Check sheet for the modelled part. Datum: model origin and axes. Units: mm. A direction names the side the tool comes from. Coordinates: 2 decimals unless noted, no trailing zeros. Write each loop counter-clockwise with the first axis right and the second up, starting at its lowest first coordinate (ties: lowest second). Pieces come first, ordered by that corner, then holes. Notation, with made-up numbers: M 31,25.5 L 84,25.5 A17 cw 84,31.5 Z; hole C -25,-32.5 d9. An arc over 180 degrees is marked long. Answer as CSV lines item,"result". Start each with the question number.
Q1. Depth check by flat-ended pin: pin 1 Ø2 at (x, z) = (6.5, 7.5) entering from +Y; pin 2 Ø8 at (x, z) = (35.5, -3) entering from +Y; pin 3 Ø1 at (y, z) = (16, 10.5) entering from +X; pin 4 Ø5 at (x, z) = (16.5, 8.5) entering from -Y. Enter the tip coordinate at first touch or a pass-through.
Q2. Access from +Z, -Z, +X, -X, +Y, -Y to the whole of each face (thin tool, end or side, straight path). Record for faces 1 (the flat face through (46, 12, -7.5)), 2 (the flat face through (3, 3, 0)), 3 (the flat face through (-5, 32, 7.5)).
Q3. Sectioned sample at A-A, the plane y = -32.5. Record the cut outline in (x, z).
Q4. Sectioned sample at D-D, the plane x = -5. Record the cut outline in (y, z).
Q5. Mould release check, pull along Z, two halves, no side actions. Record for faces 4 (the flat face through (-5, 32, -7.5)), 5 (the flat face through (0, 29, 0)), 6 (the flat face through (23, 2, -10.02)): pulls with the +Z half, pulls with the -Z half, needs draft (parallel to the pull), parting line crosses it, or undercut.
Q6. Sectioned sample at B-B, the plane z = -9. Record the cut outline in (x, y), then the cut area to 3 significant figures.
Q7. Sectioned sample at C-C, the plane y = -2.5. Record the cut outline in (x, z).
Q8. Thickness scan on line 1 along Y through (x, z) = (-4.5, 0); line 2 along Z through (x, y) = (7, -6.5); line 3 along X through (y, z) = (-22, 0). Record the ranges inside material, lowest first. Write a range as from..to.
from build123d import *

# Parameters (mm, degrees)
BOSS_EXTRUDE1_DEPTH = 15
CUT_EXTRUDE1_START  = -7
SKETCH2_W           = 20.04
SKETCH2_H           = 45
CUT_EXTRUDE1_DEPTH  = 40
SKETCH5_R           = 10.02
CUT_EXTRUDE2_DEPTH  = 40
SKETCH6_W           = 15
SKETCH6_H           = 25
CUT_EXTRUDE3_DEPTH  = 40
SKETCH7_R           = 2.5
SKETCH7_W           = 7.5
SKETCH7_H           = 15
CUT_EXTRUDE4_DEPTH  = 40
FILLET1_R           = 10


with BuildPart() as part:
    # Sketch1 → Boss-Extrude1 (new, symmetric)
    with BuildSketch(Plane.XY):
        Polygon((-10, 40), (-10, -40), (0, -40), (0, -25), (50, -25), (50, 25), (0, 25), (0, 40), align=None)
    extrude(amount=BOSS_EXTRUDE1_DEPTH, both=True)

    # Sketch2 → Cut-Extrude1 (cut)
    with BuildSketch(Plane(origin=(50, 0, 0), x_dir=(0, 0, -1), z_dir=(1, 0, 0)).offset(CUT_EXTRUDE1_START)):
        with Locations((0, 2.5)):
            Rectangle(SKETCH2_W, SKETCH2_H)
    extrude(amount=-CUT_EXTRUDE1_DEPTH, mode=Mode.SUBTRACT)

    # Sketch5 → Cut-Extrude2 (cut)
    with BuildSketch(Plane(origin=(0, -20, 0), x_dir=(1, 0, 0), z_dir=(0, 1, 0))):
        with Locations(Location((32.98, 0, 0), (0, 0, 270))):
            Circle(SKETCH5_R)
    extrude(amount=-CUT_EXTRUDE2_DEPTH, mode=Mode.SUBTRACT)

    # Sketch6 → Cut-Extrude3 (cut)
    with BuildSketch(Plane(origin=(50, 0, 0), x_dir=(0, 0, -1), z_dir=(1, 0, 0))):
        with Locations((0, 12.5)):
            Rectangle(SKETCH6_W, SKETCH6_H)
    extrude(amount=-CUT_EXTRUDE3_DEPTH, mode=Mode.SUBTRACT)

    # Sketch7 → Cut-Extrude4 (cut)
    with BuildSketch(Plane(origin=(0, 0, 0), x_dir=(0, 0, -1), z_dir=(1, 0, 0))):
        with Locations((0, 32.5)):
            Circle(SKETCH7_R)
        with Locations((0, -32.5)):
            Circle(SKETCH7_R)
        with Locations((11.25, 32.5)):
            Rectangle(SKETCH7_W, SKETCH7_H)
        with Locations((-11.25, 32.5)):
            Rectangle(SKETCH7_W, SKETCH7_H)
        with Locations((-11.25, -32.5)):
            Rectangle(SKETCH7_W, SKETCH7_H)
        with Locations((11.25, -32.5)):
            Rectangle(SKETCH7_W, SKETCH7_H)
    extrude(amount=-CUT_EXTRUDE4_DEPTH, mode=Mode.SUBTRACT)

    # Fillet1
    fillet1_edges = [part.edges().sort_by_distance(p)[0] for p in [
        (50, 0, -15),
        (50, 0, 15),
    ]]
    fillet(fillet1_edges, radius=FILLET1_R)


solid = part.part
Output:
1,pin 1,"stops at y = -20"
1,pin 2,"passes through"
1,pin 3,"stops at x = 48.66"
1,pin 4,"stops at y = -25"
2,face 1,"+X, +Y"
2,face 2,"+Y"
2,face 3,"+Z, +X, -X, +Y"
3,outline,"M -10,-7.5 L 0,-7.5 L 0,-2.5 L -10,-2.5 Z; M -10,2.5 L 0,2.5 L 0,7.5 L -10,7.5 Z"
4,outline,"M -40,-7.5 L -25,-7.5 L -25,-15 L 25,-15 L 25,-7.5 L 40,-7.5 L 40,7.5 L 25,7.5 L 25,15 L -25,15 L -25,7.5 L -40,7.5 Z; hole C -32.5,0 d5; hole C 32.5,0 d5"
5,face 4,"pulls with the -Z half"
5,face 5,"needs draft"
5,face 6,"undercut"
6,outline,"M -10,-25 L 28.58,-25 L 28.58,-20 L 3,-20 L 3,25 L -10,25 Z; M 37.38,-25 L 49.17,-25 L 49.17,25 L 43,25 L 43,-20 L 37.38,-20 Z"
6,area,"1,110 mm^2"
7,outline,"M -10,-15 L 40,-15 A10 ccw 50,-5 L 50,5 A10 ccw 40,15 L -10,15 Z; hole M 3,-10.02 L 43,-10.02 L 43,10.02 L 3,10.02 Z"
8,line 1,"y = -40..-35, -30..30, 35..40"
8,line 2,"z = -15..-10.02, 10.02..15"
8,line 3,"x = -10..22.96, 43..50"
